Input: part model. Units: mm. Frame: model coordinates. Face numbers are marked on the shaded views. Coordinates: 2 decimals unless noted, no trailing zeros. Loops run counter-clockwise (first coordinate to the right, second up) from the corner with the lowest first, then second, coordinate; pieces in that order, holes last. Notation, with made-up numbers: (51.25, -6.5) -> (56.25, -6.5) arc R27 cw to (56.25, 23.5) -> close; hole circle Ø8 at (2.25, -5.5). An arc over 180 degrees is marked (long way). Answer as a JSON object with one key per item and string values.
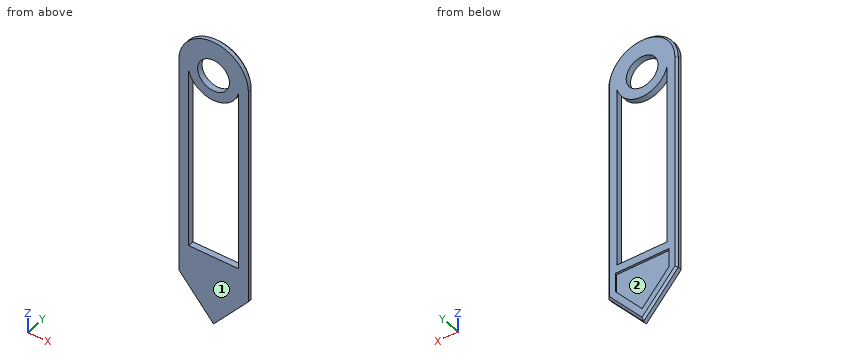
from build123d import *

# Parameters (mm, degrees)
SKETCH1_R           = 0.8
BOSS_EXTRUDE1_DEPTH = 0.3
CUT_EXTRUDE1_DEPTH  = 0.1
CHAMFER1_SIZE       = 0.1


with BuildPart() as part:
    # Sketch1 → Boss-Extrude1 (new body)
    with BuildSketch(Plane(origin=(0, 0, 0), x_dir=(1, 0, 0), z_dir=(0, 1, 0))):
        with BuildLine():
            Line((-1.75, 0), (-1.75, 11))
            Line((-1.75, 11), (0, 13))
            Line((0, 13), (1.75, 11))
            Line((1.75, 11), (1.75, 0))
            ThreePointArc((1.75, 0), (0, -1.75), (-1.75, 0))
        make_face()
        Circle(SKETCH1_R, mode=Mode.SUBTRACT)
        with BuildLine():
            Line((-1.25, 0.357071421), (-1.25, 9.5))
            Line((-1.25, 9.5), (1.25, 9.5))
            Line((1.25, 9.5), (1.25, 0.357071421))
            ThreePointArc((1.25, 0.357071421), (0, 1.3), (-1.25, 0.357071421))
        make_face(mode=Mode.SUBTRACT)
    extrude(amount=BOSS_EXTRUDE1_DEPTH)

    # Sketch2 → Cut-Extrude1 (cut)
    with BuildSketch(Plane(origin=(0, 0.3, 0), x_dir=(1, 0, 0), z_dir=(0, 1, 0))):
        Polygon((-1.35, 10.849705954), (-1.35, 9.9), (1.35, 9.9), (1.35, 10.849705954), (0, 12.392563096), align=None)
    extrude(amount=-CUT_EXTRUDE1_DEPTH, mode=Mode.SUBTRACT)

    # Chamfer1
    chamfer1_edges = [part.edges().sort_by_distance(p)[0] for p in [
        (0.875, 0.3, -12),
        (-0.875, 0.3, -12),
        (-1.75, 0.3, -5.5),
        (0, 0.3, 1.75),
        (1.75, 0.3, -5.5),
    ]]
    chamfer(chamfer1_edges, length=CHAMFER1_SIZE)


solid = part.part
1. Section query D-D (x = 0.6). Count the separate pieces of the cut face and the enclosed holes in it, plus the area to 3 significant figures.
Reply:
{"separate pieces": "3", "enclosed holes": "0", "area": "1.17 mm2"}
2. Mould query, pull axis X, two halves, no side actions, for the marked faces 1 and 2. Classes: pulls with the +X half, pulls with the -X half, needs draft (parallel to the pull), parting line crosses it, or undercut.
Reply:
{"face 1": "needs draft", "face 2": "undercut"}
3. Pin query (flat end, axial travel): P1, Ø2, axis at x = -0.5, z = -11, coming from the +Y side; P2, Ø1, axis at x = 0, z = 0, coming from the +Y side. Return the tip coordinate at first contact, or that it passes through.
Reply:
{"P1": "stops at y = 0.3", "P2": "passes through"}
4. Section query C-C (z = -11.5). Return loops of the section in (x, y), plus the area to 3 significant figures.
Reply:
{"outline": "(-1.31, 0) -> (1.31, 0) -> (1.31, 0.2) -> (1.18, 0.3) -> (0.78, 0.3) -> (0.78, 0.2) -> (-0.78, 0.2) -> (-0.78, 0.3) -> (-1.18, 0.3) -> (-1.31, 0.2) -> close", "area": "0.618 mm2"}
5. Section query B-B (y = 0.1). Return loops of the section in (x, z), plus the area to 3 significant figures.
Reply:
{"outline": "(-1.75, -11) -> (0, -13) -> (1.75, -11) -> (1.75, 0) arc R1.75 ccw to (-1.75, 0) -> close; hole (-1.25, -9.5) -> (1.25, -9.5) -> (1.25, -0.36) arc R1.3 cw to (-1.25, -0.36) -> close; hole circle Ø1.6 at (0, 0)", "area": "23.7 mm2"}
6. Line query: line 1 along X through (y, z) = (0.15, 0); line 2 along Z through (x, y) = (0.5, 0.05); line 3 along Z through (x, y) = (-0.6, 0.15). Output: solid intervals per line, ascending.
Reply:
{"line 1": "x = -1.75 to -0.8, 0.8 to 1.75", "line 2": "z = -12.43 to -9.5, -1.2 to -0.62, 0.62 to 1.68", "line 3": "z = -12.31 to -9.5, -1.15 to -0.53, 0.53 to 1.64"}
7. Section query A-A (z = -5.5). Return loops of the section in (x, y), plus the area to 3 significant figures.
Reply:
{"outline": "(-1.75, 0) -> (-1.25, 0) -> (-1.25, 0.3) -> (-1.65, 0.3) -> (-1.75, 0.2) -> close; (1.25, 0) -> (1.75, 0) -> (1.75, 0.2) -> (1.65, 0.3) -> (1.25, 0.3) -> close", "area": "0.290 mm2"}
